Here's how the part is built. I have some questions about the finished solid (model axes, mm). A direction names the side the tool comes from. Coordinates: 2 decimals unless noted, no trailing zeros. Loops run counter-clockwise (first coordinate to the right, second up) from the corner with the lowest first, then second, coordinate; pieces in that order, holes last. Notation, with made-up numbers: (13, 19) - (62, 19) arc R25 ccw to (62, 35) - close; hole circle Ø6 at (82, 84.5). An arc over 180 degrees is marked (long way). Use a Markdown table: item, result.
```python
from build123d import *

# Parameters (mm, degrees)
SKETCH3_W           = 70
SKETCH3_H           = 51.746411484
BOSS_EXTRUDE4_DEPTH = 50
SKETCH5_W           = 38.568917084
SKETCH5_H           = 32.379951318
BOSS_EXTRUDE5_DEPTH = 10
SKETCH6_R           = 8.865907929
CUT_EXTRUDE1_DEPTH  = 40
SKETCH7_R           = 2.54163754
CUT_EXTRUDE2_DEPTH  = 5
SKETCH8_R           = 4.394376148
CUT_EXTRUDE3_DEPTH  = 61


with BuildPart() as part:
    # Sketch3 → Boss-Extrude4 (new body)
    with BuildSketch(Plane(origin=(0, 0, 0), x_dir=(1, 0, 0), z_dir=(0, 1, 0))):
        Rectangle(SKETCH3_W, SKETCH3_H)
    extrude(amount=BOSS_EXTRUDE4_DEPTH)

    # Sketch5 → Boss-Extrude5 (add)
    with BuildSketch(Plane(origin=(0, 50, 0), x_dir=(1, 0, 0), z_dir=(0, 1, 0))):
        Rectangle(SKETCH5_W, SKETCH5_H)
    extrude(amount=BOSS_EXTRUDE5_DEPTH)

    # Sketch6 → Cut-Extrude1 (cut)
    with BuildSketch(Plane.XZ):
        Circle(SKETCH6_R)
    extrude(amount=-CUT_EXTRUDE1_DEPTH, mode=Mode.SUBTRACT)

    # Sketch7 → Cut-Extrude2 (cut)
    with BuildSketch(Plane.XZ.offset(-40)):
        Circle(SKETCH7_R)
    extrude(amount=-CUT_EXTRUDE2_DEPTH, mode=Mode.SUBTRACT)

    # Sketch8 → Cut-Extrude3 (cut, through all)
    with BuildSketch(Plane(origin=(0, 60, 0), x_dir=(1, 0, 0), z_dir=(0, 1, 0))):
        Circle(SKETCH8_R)
    extrude(amount=-CUT_EXTRUDE3_DEPTH, mode=Mode.SUBTRACT)


solid = part.part
```
Q1. Which directions (+Z, -Z, +X, -X, +Y, -Y) give clear straight access to the entire face, cutting with the end or side of a thin tool? Please do faces 1 (the face through (19.284, 55, 0)), 2 (the face through (0, 55, -16.19)), 3 (the face through (0, 55, 16.19)), 4 (the face through (-19.284, 55, 0)).
Check values:
| item | result |
|---|---|
| face 1 | +Z, -Z, +X, +Y |
| face 2 | -Z, +X, -X, +Y |
| face 3 | +Z, +X, -X, +Y |
| face 4 | +Z, -Z, -X, +Y |
Q2. I want a section at A-A, the plane z = 0. Write out the boundary of the cut face in (x, y), then the cut area to 3 significant figures.
Check values:
| item | result |
|---|---|
| outline | (-35, 0) - (-8.87, 0) - (-8.87, 40) - (-4.39, 40) - (-4.39, 60) - (-19.28, 60) - (-19.28, 50) - (-35, 50) - close; (4.39, 40) - (8.87, 40) - (8.87, 0) - (35, 0) - (35, 50) - (19.28, 50) - (19.28, 60) - (4.39, 60) - close |
| area | 3,000 mm^2 |
Q3. I want a section at D-D, the plane z = 11. Write out the boundary of the cut face in (x, y), then the cut area to 3 significant figures.
Check values:
| item | result |
|---|---|
| outline | (-35, 0) - (35, 0) - (35, 50) - (19.28, 50) - (19.28, 60) - (-19.28, 60) - (-19.28, 50) - (-35, 50) - close |
| area | 3,890 mm^2 |
Q4. I want a section at B-B, the plane x = 0. Write out the boundary of the cut face in (y, z).
Check values:
| item | result |
|---|---|
| outline | (0, -25.87) - (50, -25.87) - (50, -16.19) - (60, -16.19) - (60, -4.39) - (40, -4.39) - (40, -8.87) - (0, -8.87) - close; (0, 8.87) - (40, 8.87) - (40, 4.39) - (60, 4.39) - (60, 16.19) - (50, 16.19) - (50, 25.87) - (0, 25.87) - close |
Q5. Will these pins go through, and if not, where does the flat tip stop? P1, Ø5, axis at y = 57, z = 7.5, coming from the -X side; P2, Ø8, axis at x = 7.5, y = 57, coming from the -Z side; P3, Ø20.5, axis at x = 0, z = 0, coming from the +Y side; P4, Ø7, axis at x = 0, z = 0, coming from the +Y side.
Check values:
| item | result |
|---|---|
| P1 | x = -19.28 |
| P2 | z = -16.19 |
| P3 | y = 60 |
| P4 | through |
Q6. I want a section at C-C, the plane y = 46.5. Write out the boundary of the cut face in (x, z), then the cut area to 3 significant figures.
Check values:
| item | result |
|---|---|
| outline | (-35, -25.87) - (35, -25.87) - (35, 25.87) - (-35, 25.87) - close; hole circle Ø8.79 at (0, 0) |
| area | 3,560 mm^2 |
Q7. Please list where these lines run through material, in increasing order: L1, parallel to X at y = 52.5, z = 0; L2, parallel to Z at x = 0, y = 22; L3, parallel to Z at x = 0, y = 52. Write a range as from..to.
Check values:
| item | result |
|---|---|
| L1 | -19.28..-4.39, 4.39..19.28 |
| L2 | -25.87..-8.87, 8.87..25.87 |
| L3 | -16.19..-4.39, 4.39..16.19 |
Q8. If we mould it in two halves opening along Z, with no side actions, what happens to faces 5 (the face through (0, 25, 25.873)), 6 (the face through (-6.535, 19.72, 5.992)), 7 (the face through (0, 25, -25.873))? For each: pulls with the +Z half, pulls with the -Z half, needs draft (parallel to the pull), parting line crosses it, or undercut.
Check values:
| item | result |
|---|---|
| face 5 | pulls with the +Z half |
| face 6 | undercut |
| face 7 | pulls with the -Z half |
